For this review, use the dimensioned drawing (mm, ordinates from the lowest corner) and the shaded views. A direction names the side the tool comes from. Give positions to 0.01 mm unless a question says otherwise; leave off trailing zeros. Order: outer loops, then holes, each group sorted by start corner. A loop starts at its lowest first (then second) coordinate and runs counter-clockwise, first axis right, second up.
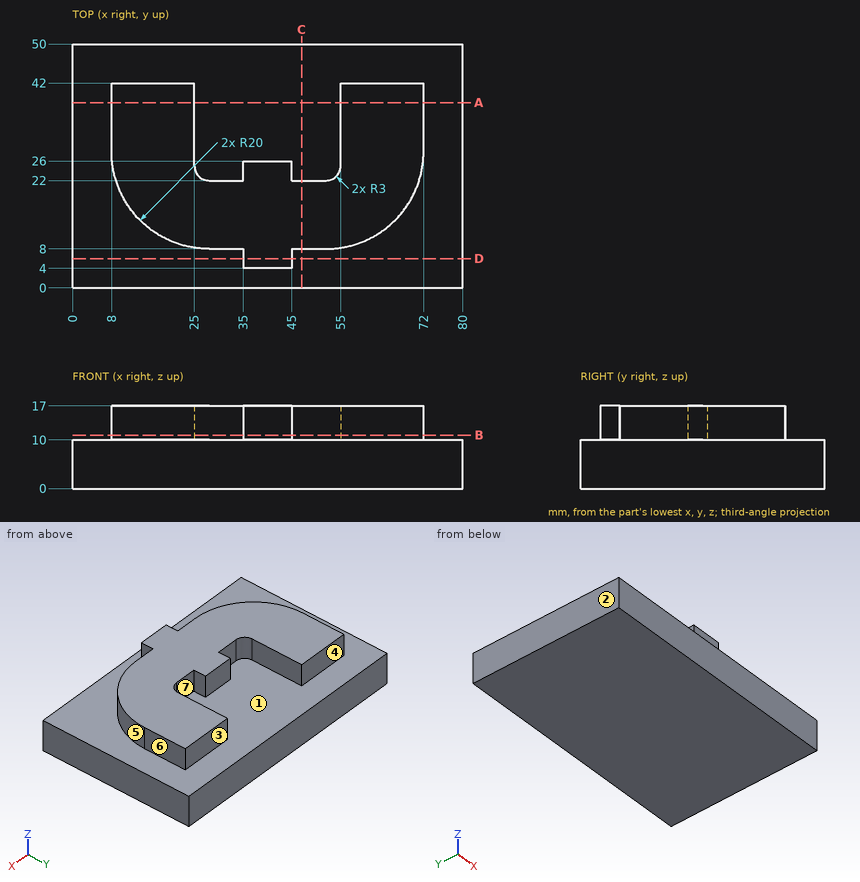
1. For line 1 along X through (y, z) = (33.5, 15); line 2 along Z through (x, y) = (72, 15); line 3 along X through (y, z) = (23.5, 15.5), list the stretches that pass through material, from the lowest coordinate up.
Recorded:
line 1: x = 8 to 25, 55 to 72
line 2: z = 0 to 10
line 3: x = 8.51 to 25.4, 35 to 45, 54.6 to 71.49
2. For pin 1 (3.5 mm diameter, centred on x = 39, z = 12.5, fed in from -Y); pin 2 (3.5 mm diameter, centred on x = 63.5, z = 15, fed in from +Y); pin 3 (1.2 mm diameter, centred on y = 23.5, z = 12.5, fed in from +X), all flat-tipped, find the tip position at first contact; note any pin that passes through.
Recorded:
pin 1: stops at y = 4
pin 2: stops at y = 42
pin 3: stops at x = 71.62
3. Machinability: for the marked faces 4, 5, 6 and 7, which of the approach directions +Z, -Z, +X, -X, +Y, -Y give a long, thin tool a straight path to every point of the face, cutting with its end or side? Answer none if there is none.
Recorded:
face 4: +Z, +X, -X, +Y
face 5: +Z, +X, -Y
face 6: +Z, +X, +Y, -Y
face 7: +Z, +Y
4. Draft analysis for pull direction X (two halves, no side actions). For the marked faces 1, 2 and 3, state which applies: pulls with the +X half, pulls with the -X half, needs draft (parallel to the pull), parting line crosses it, or undercut.
Recorded:
face 1: undercut
face 2: pulls with the -X half
face 3: needs draft
5. Take a section at A-A (y = 38). State the section outline as (x, z) points, then the cut area to 3 significant figures.
Recorded:
outline: (0, 0) - (80, 0) - (80, 10) - (72, 10) - (72, 17) - (55, 17) - (55, 10) - (25, 10) - (25, 17) - (8, 17) - (8, 10) - (0, 10) - close
area: 1,040 mm2
6. Take a section at B-B (z = 11). State the section outline as (x, y) points.
Recorded:
outline: (8, 28) arc R20 ccw to (28, 8) - (35, 8) - (35, 4) - (45, 4) - (45, 8) - (52, 8) arc R20 ccw to (72, 28) - (72, 42) - (55, 42) - (55, 25) arc R3 cw to (52, 22) - (45, 22) - (45, 26) - (35, 26) - (35, 22) - (28, 22) arc R3 cw to (25, 25) - (25, 42) - (8, 42) - close
7. Take a section at D-D (y = 6). State the section outline as (x, z) points, then the cut area to 3 significant figures.
Recorded:
outline: (0, 0) - (80, 0) - (80, 10) - (45, 10) - (45, 17) - (35, 17) - (35, 10) - (0, 10) - close
area: 870 mm2
8. Take a section at C-C (x = 47). State the section outline as (y, z) points.
Recorded:
outline: (0, 0) - (50, 0) - (50, 10) - (22, 10) - (22, 17) - (8, 17) - (8, 10) - (0, 10) - close
